```python
from build123d import *

# Parameters (mm, degrees)
SKETCH1_R           = 11.176
BOSS_EXTRUDE1_DEPTH = 3.81
SKETCH2_W           = 41.91
SKETCH2_H           = 1.27
BOSS_EXTRUDE2_DEPTH = 1.016
BOSS_EXTRUDE4_START = 2.286
SKETCH4_R           = 13.716
SKETCH4_R_2         = 11.176
BOSS_EXTRUDE4_DEPTH = 2.286


with BuildPart() as part:
    # Sketch1 → Boss-Extrude1 (new body)
    with BuildSketch(Plane.XY):
        with BuildLine():
            Line((20.955, -25.4), (20.955, -21.59))
            Line((20.955, -21.59), (-20.955, -21.59))
            Line((-20.955, -21.59), (-20.955, 21.59))
            Line((-20.955, 21.59), (20.955, 21.59))
            Line((20.955, 21.59), (20.955, 25.4))
            Line((20.955, 25.4), (46.355, 25.4))
            ThreePointArc((46.355, 25.4), (71.755, 0), (46.355, -25.4))
            Line((46.355, -25.4), (20.955, -25.4))
        make_face()
        with Locations(Location((53.975, 0, 0), (0, 0, 180))):
            Circle(SKETCH1_R, mode=Mode.SUBTRACT)
    extrude(amount=BOSS_EXTRUDE1_DEPTH)

    # Sketch2 → Boss-Extrude2 (add)
    with BuildSketch(Plane.XZ.offset(21.59)):
        with Locations((0, 1.905)):
            Rectangle(SKETCH2_W, SKETCH2_H)
    boss_extrude2 = extrude(amount=BOSS_EXTRUDE2_DEPTH)

    # Mirror1: Boss-Extrude2 across plane
    add(boss_extrude2.mirror(Plane.ZX))

    # Sketch4 → Boss-Extrude4 (add)
    with BuildSketch(Plane(origin=(0, 0, 0), x_dir=(-1, 0, 0), z_dir=(0, 0, -1)).offset(BOSS_EXTRUDE4_START)):
        with Locations((-53.975, 0)):
            Circle(SKETCH4_R)
        with Locations((-53.975, 0)):
            Circle(SKETCH4_R_2, mode=Mode.SUBTRACT)
    extrude(amount=-BOSS_EXTRUDE4_DEPTH)


solid = part.part
```
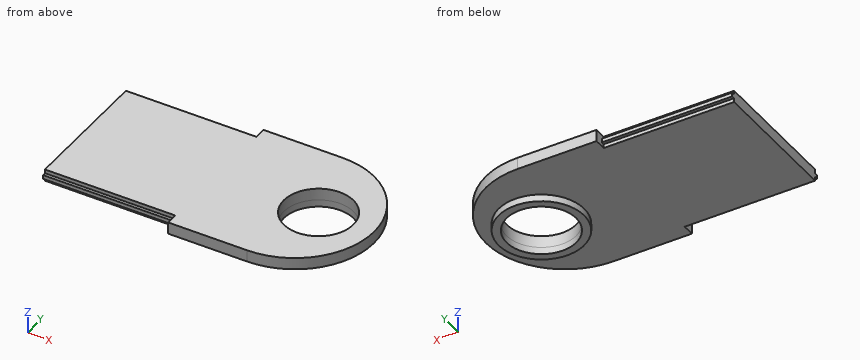
Geometry: final body of the model. Coordinates: model frame, mm. Round coordinates to 2 decimals unless told otherwise and drop trailing zeros. Write each loop counter-clockwise with the first axis right and the second up, starting at its lowest first coordinate (ties: lowest second). Pieces come first, ordered by that corner, then holes.
Item 1: Section query B-B (x = 53). Return loops of the section in (y, z).
Item 2: Pin query (flat end, axial travel): P1, Ø0.5, axis at x = -7.5, y = -22, coming from the -Z side; P2, Ø1.5, axis at x = 12.5, y = 18.5, coming from the -Z side; P3, Ø1, axis at x = -7, z = 3.5, coming from the +Y side. Return the tip coordinate at first contact, or that it passes through.
Item 3: Section query A-A (y = 0). Return loops of the section in (x, z) (3 decimals), plus the area to 3 significant figures.
Item 4: Material intervals for L1, parallel to Z at x = 46, y = 14; L2, parallel to Y at x = 4, z = 2.5; L3, parallel to Y at x = 50, z = 3.5, sorted ascending.
Item 5: Section query D-D (z = -1.25). Return loops of the section in (x, y) (3 decimals), plus the area to 3 significant figures.
Item 6: Section query C-C (x = 16). Return loops of the section in (y, z).
Completed:
1. outline: (-24.52, 0) - (-13.68, 0) - (-13.68, -2.29) - (-11.13, -2.29) - (-11.13, 3.81) - (-24.52, 3.81) - close; (11.13, -2.29) - (13.68, -2.29) - (13.68, 0) - (24.52, 0) - (24.52, 3.81) - (11.13, 3.81) - close
2. P1: stops at z = 1.27
2. P2: stops at z = 0
2. P3: stops at y = 21.59
3. outline: (-20.955, 0) - (40.259, 0) - (40.259, -2.286) - (42.799, -2.286) - (42.799, 3.81) - (-20.955, 3.81) - close; (65.151, -2.286) - (67.691, -2.286) - (67.691, 0) - (71.755, 0) - (71.755, 3.81) - (65.151, 3.81) - close
3. area: 280 mm2
4. L1: z = 0 to 3.81
4. L2: y = -22.61 to 22.61
4. L3: y = -25.14 to -10.45, 10.45 to 25.14
5. outline: circle Ø27.432 at (53.975, 0); hole circle Ø22.352 at (53.975, 0)
5. area: 199 mm2
6. outline: (-22.61, 1.27) - (-21.59, 1.27) - (-21.59, 0) - (21.59, 0) - (21.59, 1.27) - (22.61, 1.27) - (22.61, 2.54) - (21.59, 2.54) - (21.59, 3.81) - (-21.59, 3.81) - (-21.59, 2.54) - (-22.61, 2.54) - close
